Autodesk Inventor part; units mm, degrees
ref_plane "YZ Plane" through (0, 0, 0) normal (1, 0, 0) x (0, 1, 0)
ref_plane "XZ Plane" through (0, 0, 0) normal (0, 1, 0) x (-1, 0, 0)
ref_plane "XY Plane" through (0, 0, 0) normal (0, 0, 1) x (1, 0, 0)
sketch "Sketch1" plane through (0, 0, 0) normal (0, 1, 0) x (-1, 0, 0)
  line L0 (0, 0) -> (190.5, 0)
  line L1 (190.5, 0) -> (190.5, -215.9)
  line L2 (190.5, -215.9) -> (0, -215.9)
  line L3 (0, -215.9) -> (0, 0)
  dimension "d0" = 215.9
  dimension "d1" = 190.5
extrude "Extrusion1" add sketch "Sketch1" along normal blind 12.7
sketch "Sketch2" plane through (0, 0, 0) normal (0, -1, 0) x (1, 0, 0)
  line L0 (-190.5, 0) -> (0, 0) construction
  line L1 (0, -215.9) -> (-190.5, -215.9) construction
  line L2 (0, 0) -> (-190.5, 0)
  line L3 (-190.5, 0) -> (-190.5, -215.9) construction
  line L4 (-190.5, -215.9) -> (0, -215.9)
  line L5 (0, -215.9) -> (0, 0) construction
  line L6 (-184.15, -209.55) -> (-184.15, -6.35)
  line L7 (-184.15, -6.35) -> (-6.35, -6.35)
  line L8 (-6.35, -6.35) -> (-6.35, -209.55)
  line L9 (-6.35, -209.55) -> (-184.15, -209.55)
  line L10 (-177.8, -203.2) -> (-12.7, -203.2)
  line L11 (-12.7, -12.7) -> (-63.5, -12.7)
  line L12 (-63.5, -12.7) -> (-63.5, -120.65)
  line L13 (-63.5, -120.65) -> (-12.7, -120.65)
  line L14 (-12.7, -120.65) -> (-12.7, -12.7)
  line L15 (-69.85, -120.65) -> (-69.85, -12.7)
  line L16 (-127, -6.35) -> (-6.35, -6.35)
  line L17 (-6.35, -6.35) -> (-6.35, -127)
  line L18 (-12.7, -127) -> (-127, -127)
  line L19 (-127, -127) -> (-177.8, -127)
  line L20 (-69.85, -120.65) -> (-177.8, -120.65)
  line L21 (-12.7, -12.7) -> (-63.5, -12.7)
  line L22 (-69.85, -12.7) -> (-177.8, -12.7)
  line L23 (-12.7, -203.2) -> (-12.7, -127)
  line L24 (-12.7, -120.65) -> (-12.7, -12.7)
  line L25 (-177.8, -12.7) -> (-177.8, -120.65)
  line L26 (-177.8, -127) -> (-177.8, -203.2)
  dimension "d4" = 6.35
  dimension "d8" = 6.35
  dimension "d11" = 107.95
  dimension "d12" = 107.95
extrude "Extrusion2" cut sketch "Sketch2" against normal blind 6.35
properties part number "RSX Top" material "Aluminum 6061"
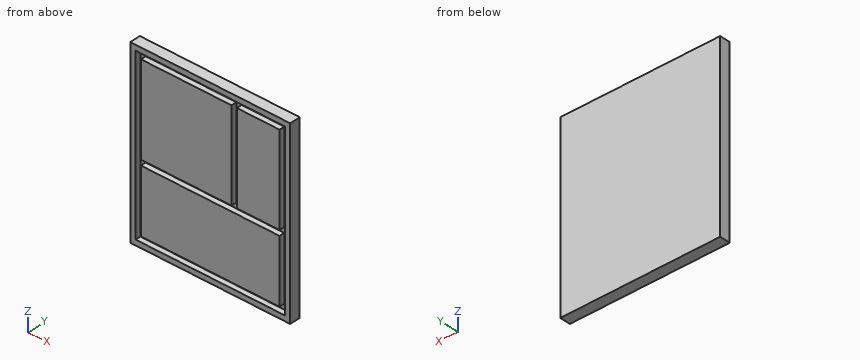
Work out the finished part from the listing and answer in its coordinate system (mm). Coordinates: 2 decimals unless noted, no trailing zeros. Write each loop counter-clockwise with the first axis right and the second up, starting at its lowest first coordinate (ties: lowest second). Pieces come first, ordered by that corner, then holes.
Q1. A cutting plane is placed at A-A, the plane y = 4. Give the vertices of the cut face in (x, z), then the cut area to 3 significant figures.
Q2. Find the intervals of material crossed by line 1 (Z direction, x = -26.5, y = 4); line 2 (X direction, y = 1, z = -158.5); line 3 (X direction, y = 4.75, z = -98), in increasing order.
Q3. A cutting plane is placed at D-D, the plane z = -56.5. Give the vertices of the cut face in (x, y), then the cut area to 3 significant figures.
Q4. A cutting plane is placed at C-C, the plane x = -67. Give the vertices of the cut face in (y, z).
Q5. A cutting plane is placed at B-B, the plane z = -134. Give the vertices of the cut face in (x, y).
Findings below:
1. outline: (-190.5, -215.9) - (0, -215.9) - (0, 0) - (-190.5, 0) - close; (-177.8, -203.2) - (-12.7, -203.2) - (-12.7, -127) - (-177.8, -127) - close; (-177.8, -120.65) - (-69.85, -120.65) - (-69.85, -12.7) - (-177.8, -12.7) - close; (-63.5, -120.65) - (-12.7, -120.65) - (-12.7, -12.7) - (-63.5, -12.7) - close; hole (-184.15, -209.55) - (-6.35, -209.55) - (-6.35, -6.35) - (-184.15, -6.35) - close
1. area: 34,700 mm2
2. line 1: z = -215.9 to -209.55, -203.2 to -127, -120.65 to -12.7, -6.35 to 0
2. line 2: x = -190.5 to -184.15, -177.8 to -12.7, -6.35 to 0
2. line 3: x = -190.5 to -184.15, -177.8 to -69.85, -63.5 to -12.7, -6.35 to 0
3. outline: (-190.5, 0) - (-184.15, 0) - (-184.15, 6.35) - (-177.8, 6.35) - (-177.8, 0) - (-69.85, 0) - (-69.85, 6.35) - (-63.5, 6.35) - (-63.5, 0) - (-12.7, 0) - (-12.7, 6.35) - (-6.35, 6.35) - (-6.35, 0) - (0, 0) - (0, 12.7) - (-190.5, 12.7) - close
3. area: 2,300 mm2
4. outline: (0, -215.9) - (12.7, -215.9) - (12.7, 0) - (0, 0) - (0, -6.35) - (6.35, -6.35) - (6.35, -127) - (0, -127) - (0, -203.2) - (6.35, -203.2) - (6.35, -209.55) - (0, -209.55) - close
5. outline: (-190.5, 0) - (-184.15, 0) - (-184.15, 6.35) - (-177.8, 6.35) - (-177.8, 0) - (-12.7, 0) - (-12.7, 6.35) - (-6.35, 6.35) - (-6.35, 0) - (0, 0) - (0, 12.7) - (-190.5, 12.7) - close
